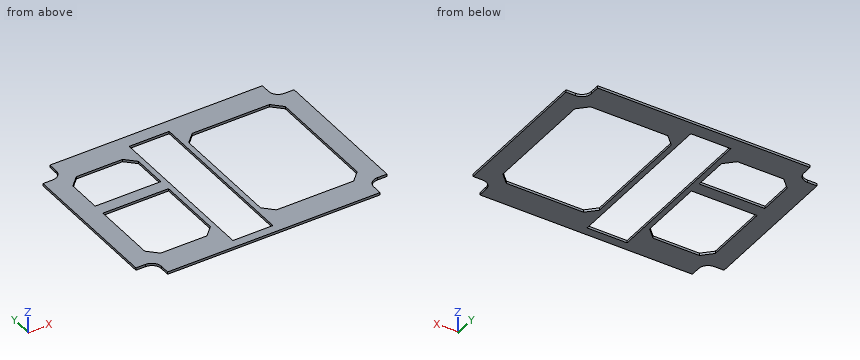
from build123d import *

# Parameters (mm, degrees)
SKETCH1_W           = 20.32
SKETCH1_H           = 100.33
BOSS_EXTRUDE1_DEPTH = 1.5875
SKETCH2_W           = 26.32
SKETCH2_H           = 106.33
CUT_EXTRUDE1_DEPTH  = 2.5875


with BuildPart() as part:
    # Sketch1 → Boss-Extrude1 (new body)
    with BuildSketch(Plane.XY):
        with BuildLine():
            Line((0, -12.7), (-6.35, -12.7))
            ThreePointArc((-6.35, -12.7), (-10.840128061, -10.840128061), (-12.7, -6.35))
            Line((-12.7, -6.35), (-12.7, 0))
            Line((-12.7, 0), (-152.4, 0))
            Line((-152.4, 0), (-152.4, -6.35))
            ThreePointArc((-152.4, -6.35), (-154.259871939, -10.840128061), (-158.75, -12.7))
            Line((-158.75, -12.7), (-165.1, -12.7))
            Line((-165.1, -12.7), (-165.1, -107.95))
            Line((-165.1, -107.95), (-158.75, -107.95))
            ThreePointArc((-158.75, -107.95), (-154.259871939, -109.809871939), (-152.4, -114.3))
            Line((-152.4, -114.3), (-152.4, -120.65))
            Line((-152.4, -120.65), (-12.7, -120.65))
            Line((-12.7, -120.65), (-12.7, -114.3))
            ThreePointArc((-12.7, -114.3), (-10.840128061, -109.809871939), (-6.35, -107.95))
            Line((-6.35, -107.95), (0, -107.95))
            Line((0, -107.95), (0, -12.7))
        make_face()
        with Locations((-92.71, -61.849)):
            Rectangle(SKETCH1_W, SKETCH1_H, mode=Mode.SUBTRACT)
        Polygon((-19.05, -17.145), (-69.85, -17.145), (-76.2, -23.495), (-76.2, -97.155), (-69.85, -103.505), (-19.05, -103.505), (-12.7, -97.155), (-12.7, -23.495), align=None, mode=Mode.SUBTRACT)
        Polygon((-152.4, -23.495), (-152.4, -46.355), (-109.22, -46.355), (-109.22, -23.495), (-115.57, -17.145), (-146.05, -17.145), align=None, mode=Mode.SUBTRACT)
        Polygon((-109.22, -97.155), (-109.22, -54.2925), (-152.4, -54.2925), (-152.4, -97.155), (-146.05, -103.505), (-115.57, -103.505), align=None, mode=Mode.SUBTRACT)
    extrude(amount=BOSS_EXTRUDE1_DEPTH)

    # Sketch2 → Cut-Extrude1 (cut, through all)
    with BuildSketch(Plane(origin=(0, 0, 0), x_dir=(-1, 0, 0), z_dir=(0, 0, -1))):
        with Locations((92.71, -61.849)):
            Rectangle(SKETCH2_W, SKETCH2_H)
    extrude(amount=-CUT_EXTRUDE1_DEPTH, mode=Mode.SUBTRACT)


solid = part.part
Build history of the part. All positions in model axes, mm. Round coordinates to 2 decimals unless told otherwise and drop trailing zeros. Write each loop counter-clockwise with the first axis right and the second up, starting at its lowest first coordinate (ties: lowest second). Pieces come first, ordered by that corner, then holes. Notation, with made-up numbers: (59.25, 84) - (85.25, 84) arc R13 cw to (85.25, 96) - close; hole circle Ø10 at (22.5, -38.5). An arc over 180 degrees is marked (long way). Use CSV: the item, a comma, the result in double quotes.
(1) Band-saw the part on C-C (x = -85). Write the cut outline in (y, z), plus the area to 3 significant figures.
Response:
outline,"(-120.65, 0) - (-115.01, 0) - (-115.01, 1.59) - (-120.65, 1.59) - close; (-8.68, 0) - (0, 0) - (0, 1.59) - (-8.68, 1.59) - close"
area,"22.7 mm²"
(2) Band-saw the part on A-A (x = -117.5). Give the number of separate pieces and of enclosed holes in the cut face, plus the area to 3 significant figures.
Response:
separate pieces,"3"
enclosed holes,"0"
area,"67.0 mm²"
(3) Band-saw the part on B-B (y = -90.5). Write the cut outline in (x, z), plus the area to 3 significant figures.
Response:
outline,"(-165.1, 0) - (-152.4, 0) - (-152.4, 1.59) - (-165.1, 1.59) - close; (-109.22, 0) - (-105.87, 0) - (-105.87, 1.59) - (-109.22, 1.59) - close; (-79.55, 0) - (-76.2, 0) - (-76.2, 1.59) - (-79.55, 1.59) - close; (-12.7, 0) - (0, 0) - (0, 1.59) - (-12.7, 1.59) - close"
area,"51.0 mm²"
(4) Wall check: line 1 (X direction, y = -94.5, z = 1.4); line 2 (X direction, y = -54, z = 1.3); line 3 (X direction, y = -102, z = 1.05) (3 decimals). Give the ranges that are in metal, low to high.
Response:
line 1,"-165.1 to -152.4, -109.22 to -105.87, -79.55 to -76.2, -12.7 to 0"
line 2,"-165.1 to -105.87, -79.55 to -76.2, -12.7 to 0"
line 3,"-165.1 to -147.555, -114.065 to -105.87, -79.55 to -71.355, -17.545 to 0"
(5) Pin check, flat tip, straight feed: P1, Ø0.8, axis at x = -163.5, z = 1, coming from the -Y side. Stop position of the tip, or through.
Response:
P1,"y = -107.95"
